```python
from build123d import *

# Parameters (mm, degrees)
SKETCH_1_W               = 75
SKETCH_1_H               = 16
SKETCH_1_R               = 4
EXTRUDE_1_DEPTH          = 2.5
SKETCH_3_W               = 75
SKETCH_3_H               = 5
EXTRUDE_2_DEPTH          = 60
CUT_EXTRUDE_1_REACH      = 89.199
SKETCH_4_R               = 2
SKETCH_5_W               = 75
SKETCH_5_H               = 5
EXTRUDE_3_DEPTH          = 60
SKETCH_6_W               = 10
SKETCH_6_H               = 16
EXTRUDE_4_DEPTH          = 22
CUT_EXTRUDE_2_DEPTH      = 113.985345572
CUT_EXTRUDE_2_DEPTH_BACK = 113.985345572
SKETCH_7_R               = 4
CHAMFER_1_SIZE           = 4


with BuildPart() as part:
    # 草图1 → 凸台-拉伸1 (new body)
    with BuildSketch(Plane(origin=(0, 0, 0), x_dir=(1, 0, 0), z_dir=(0, 1, 0))):
        with Locations((24.811158798, 1.43319531)):
            Rectangle(SKETCH_1_W, SKETCH_1_H)
        with Locations(Location((-7.188841202, 3.93319531, 0), (0, 0, 270))):
            Circle(SKETCH_1_R, mode=Mode.SUBTRACT)
        with Locations(Location((56.811158798, 3.93319531, 0), (0, 0, 270))):
            Circle(SKETCH_1_R, mode=Mode.SUBTRACT)
    extrude(amount=-EXTRUDE_1_DEPTH)

    # 草图3 → 凸台-拉伸2 (add)
    with BuildSketch(Plane(origin=(0, 0, 0), x_dir=(1, 0, 0), z_dir=(0, 1, 0))):
        with Locations((24.811158798, -4.06680469)):
            Rectangle(SKETCH_3_W, SKETCH_3_H)
    extrude(amount=EXTRUDE_2_DEPTH)

    # 草图4 → 切除-拉伸1 (cut, up to next)
    with BuildSketch(Plane(origin=(0, 0, 1.56680469), x_dir=(-1, 0, 0), z_dir=(0, 0, -1)), mode=Mode.PRIVATE) as cut_extrude_1_sk1:
        with Locations((-9.811158798, 13)):
            Circle(SKETCH_4_R)
    cut_extrude_1_tool1 = extrude(cut_extrude_1_sk1.sketch, amount=-CUT_EXTRUDE_1_REACH, mode=Mode.PRIVATE) & part.part
    # 草图4 → 切除-拉伸1 (cut, up to next)
    with BuildSketch(Plane(origin=(0, 0, 1.56680469), x_dir=(-1, 0, 0), z_dir=(0, 0, -1)), mode=Mode.PRIVATE) as cut_extrude_1_sk2:
        with Locations((-9.811158798, 41)):
            Circle(SKETCH_4_R)
    cut_extrude_1_tool2 = extrude(cut_extrude_1_sk2.sketch, amount=-CUT_EXTRUDE_1_REACH, mode=Mode.PRIVATE) & part.part
    # 草图4 → 切除-拉伸1 (cut, up to next)
    with BuildSketch(Plane(origin=(0, 0, 1.56680469), x_dir=(-1, 0, 0), z_dir=(0, 0, -1)), mode=Mode.PRIVATE) as cut_extrude_1_sk3:
        with Locations((-39.811158798, 41)):
            Circle(SKETCH_4_R)
    cut_extrude_1_tool3 = extrude(cut_extrude_1_sk3.sketch, amount=-CUT_EXTRUDE_1_REACH, mode=Mode.PRIVATE) & part.part
    # 草图4 → 切除-拉伸1 (cut, up to next)
    with BuildSketch(Plane(origin=(0, 0, 1.56680469), x_dir=(-1, 0, 0), z_dir=(0, 0, -1)), mode=Mode.PRIVATE) as cut_extrude_1_sk4:
        with Locations((-39.811158798, 13)):
            Circle(SKETCH_4_R)
    cut_extrude_1_tool4 = extrude(cut_extrude_1_sk4.sketch, amount=-CUT_EXTRUDE_1_REACH, mode=Mode.PRIVATE) & part.part
    add(cut_extrude_1_tool1.solids().sort_by_distance((9.811159, 13, 1.566805))[0], mode=Mode.SUBTRACT)
    add(cut_extrude_1_tool2.solids().sort_by_distance((9.811159, 41, 1.566805))[0], mode=Mode.SUBTRACT)
    add(cut_extrude_1_tool3.solids().sort_by_distance((39.811159, 41, 1.566805))[0], mode=Mode.SUBTRACT)
    add(cut_extrude_1_tool4.solids().sort_by_distance((39.811159, 13, 1.566805))[0], mode=Mode.SUBTRACT)

    # 草图5 → 凸台-拉伸3 (add)
    with BuildSketch(Plane(origin=(0, 0, 1.56680469), x_dir=(-1, 0, 0), z_dir=(0, 0, -1))):
        with Locations((-24.811158798, 57.5)):
            Rectangle(SKETCH_5_W, SKETCH_5_H)
    extrude(amount=EXTRUDE_3_DEPTH)

    # 草图6 → 凸台-拉伸4 (add)
    with BuildSketch(Plane.XZ.offset(-55)):
        with Locations((40.811158798, -28.43319531)):
            Rectangle(SKETCH_6_W, SKETCH_6_H)
        with Locations((8.811158798, -28.43319531)):
            Rectangle(SKETCH_6_W, SKETCH_6_H)
    extrude(amount=-EXTRUDE_4_DEPTH)

    # 草图7 → 切除-拉伸2 (cut, two sides: drawn at the far end of the back side and taken through both)
    with BuildSketch(Plane(origin=(45.811158798, 0, 0), x_dir=(0, 0, -1), z_dir=(1, 0, 0)).offset(-CUT_EXTRUDE_2_DEPTH_BACK)):
        with Locations((28.43319531, 71)):
            Circle(SKETCH_7_R)
    extrude(amount=CUT_EXTRUDE_2_DEPTH + CUT_EXTRUDE_2_DEPTH_BACK, mode=Mode.SUBTRACT)

    # 倒角1
    chamfer_1_edges = [part.edges().sort_by_distance(p)[0] for p in [
        (40.811158798, 77, -20.43319531),
        (40.811158798, 77, -36.43319531),
        (8.811158798, 77, -36.43319531),
        (8.811158798, 77, -20.43319531),
    ]]
    chamfer(chamfer_1_edges, length=CHAMFER_1_SIZE)


solid = part.part
```
The model under review builds one solid part; all positions refer to its coordinate system, in mm. A direction names the side the tool comes from. Give positions to 0.01 mm unless a question says otherwise; leave off trailing zeros. Loops run counter-clockwise (first coordinate to the right, second up) from the corner with the lowest first, then second, coordinate; pieces in that order, holes last. Notation, with made-up numbers: (19.25, -37) -> (74.25, -37) arc R25 ccw to (74.25, -19) -> close; hole circle Ø6 at (85.5, 71.5). An arc over 180 degrees is marked (long way). Use CSV: the item, a comma, the result in double quotes.
1. Machinability: for faces 4 (the face through (24, 55, -28)), 5 (the face through (13.811, 66, -29)), 6 (the face through (9, 66, -36.433)), 7 (the face through (45.811, 66, -29)), which of the approach directions +Z, -Z, +X, -X, +Y, -Y give a long, thin tool a straight path to every point of the face, cutting with its end or side? Answer none if there is none.
Result:
face 4,"-Z, +X, -X"
face 5,"+Z, -Z, +Y"
face 6,"-Z, +X, -X, +Y"
face 7,"+Z, -Z, +X, +Y"
2. For P1, Ø5, axis at x = 33, z = -17.5, coming from the -Y side; P2, Ø12, axis at y = 39.5, z = -4.5, coming from the -X side; P3, Ø9, axis at y = 71, z = -28.43, coming from the -X side; P4, Ø3, axis at x = 7, y = 65.5, coming from the +Z side, all flat-tipped, find the tip position at first contact; note any pin that passes through.
Result:
P1,"stops at y = 55"
P2,"passes through"
P3,"stops at x = 3.81"
P4,"stops at z = -20.43"
3. Consider section A-A, the plane y = 71. Write out the cut boundary in (x, z).
Result:
outline,"(3.81, -36.43) -> (13.81, -36.43) -> (13.81, -32.43) -> (3.81, -32.43) -> close; (3.81, -24.43) -> (13.81, -24.43) -> (13.81, -20.43) -> (3.81, -20.43) -> close; (35.81, -36.43) -> (45.81, -36.43) -> (45.81, -32.43) -> (35.81, -32.43) -> close; (35.81, -24.43) -> (45.81, -24.43) -> (45.81, -20.43) -> (35.81, -20.43) -> close"
4. The part is to be moulded in two halves that separate along Z. For faces 1 (the face through (8.741, 67.095, -27.566)), 2 (the face through (24, 0, -4)), 3 (the face through (9, 66, -20.433)), say which applies: +Z half, -Z half, draft (parallel to the pull), parting line (faces both ways), or undercut.
Result:
face 1,"undercut"
face 2,"draft"
face 3,"+Z half"
5. Consider section D-D, the plane y = 13. Write out the cut boundary in (x, z).
Result:
outline,"(-12.69, 1.57) -> (7.81, 1.57) -> (7.81, 6.57) -> (-12.69, 6.57) -> close; (11.81, 1.57) -> (37.81, 1.57) -> (37.81, 6.57) -> (11.81, 6.57) -> close; (41.81, 1.57) -> (62.31, 1.57) -> (62.31, 6.57) -> (41.81, 6.57) -> close"
6. Consider section B-B, the plane x = 25. Write out the cut boundary in (y, z).
Result:
outline,"(-2.5, -9.43) -> (0, -9.43) -> (0, 1.57) -> (55, 1.57) -> (55, -58.43) -> (60, -58.43) -> (60, 6.57) -> (-2.5, 6.57) -> close"
7. Consider section C-C, the plane z = -2.5. Write out the cut boundary in (x, y).
Result:
outline,"(-12.69, -2.5) -> (-10.92, -2.5) -> (-10.92, 0) -> (-12.69, 0) -> close; (-12.69, 55) -> (62.31, 55) -> (62.31, 60) -> (-12.69, 60) -> close; (-3.45, -2.5) -> (53.08, -2.5) -> (53.08, 0) -> (-3.45, 0) -> close; (60.55, -2.5) -> (62.31, -2.5) -> (62.31, 0) -> (60.55, 0) -> close"
8. To check wall thickness, follow probe 1 along Z at (x, y) = (40, 71); probe 2 along X at (y, z) = (62.5, -24); probe 3 along Y at (x, z) = (35, 1.5). State the ranges of each line that lie inside material, in increasing order. Write a range as from..to.
Result:
probe 1,"z = -36.43..-32.43, -24.43..-20.43"
probe 2,"x = 3.81..13.81, 35.81..45.81"
probe 3,"y = -2.5..0, 55..60"
